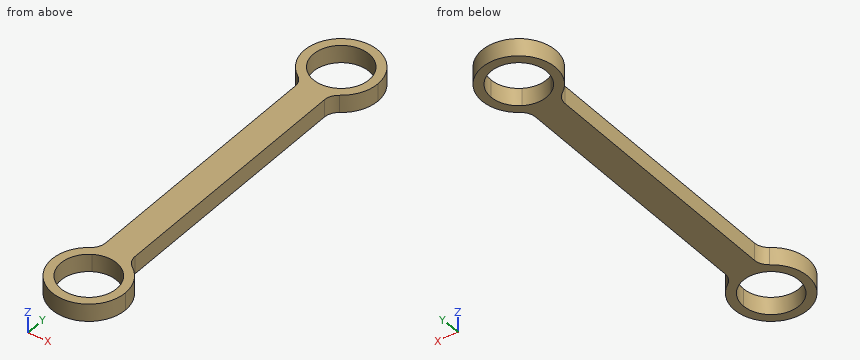
from build123d import *

# Parameters (mm, degrees)
SALIENTE_EXTRUIR1_DEPTH = 6
REDONDEO1_R             = 5


with BuildPart() as part:
    # Croquis1 → Saliente-Extruir1 (new body)
    with BuildSketch(Plane.XY):
        with BuildLine():
            ThreePointArc((-5, 103.543560763), (0, 102.5), (5, 103.543560763))
            Line((5, 103.543560763), (5, 106.922252789))
            ThreePointArc((5, 106.922252789), (0, 105.5), (-5, 106.922252789))
            Line((-5, 106.922252789), (-5, 103.543560763))
        make_face()
        with BuildLine():
            Line((5, 106.922252789), (5, 103.543560763))
            ThreePointArc((5, 103.543560763), (10.458250332, 108.153468031), (12.5, 115))
            ThreePointArc((12.5, 115), (-6.846531969, 125.458250332), (-5, 103.543560763))
            Line((-5, 103.543560763), (-5, 106.922252789))
            ThreePointArc((-5, 106.922252789), (-4.623310502, 123.299096336), (9.5, 115))
            ThreePointArc((9.5, 115), (8.299096336, 110.376689498), (5, 106.922252789))
        make_face()
        with BuildLine():
            ThreePointArc((-5, 11.456439237), (0, 12.5), (5, 11.456439237))
            Line((5, 11.456439237), (5, 103.543560763))
            ThreePointArc((5, 103.543560763), (0, 102.5), (-5, 103.543560763))
            Line((-5, 103.543560763), (-5, 11.456439237))
        make_face()
        with BuildLine():
            ThreePointArc((-5, 8.077747211), (0, 9.5), (5, 8.077747211))
            Line((5, 8.077747211), (5, 11.456439237))
            ThreePointArc((5, 11.456439237), (0, 12.5), (-5, 11.456439237))
            Line((-5, 11.456439237), (-5, 8.077747211))
        make_face()
        with BuildLine():
            Line((5, 11.456439237), (5, 8.077747211))
            ThreePointArc((5, 8.077747211), (8.299096336, 4.623310502), (9.5, 0))
            ThreePointArc((9.5, 0), (-4.623310502, -8.299096336), (-5, 8.077747211))
            Line((-5, 8.077747211), (-5, 11.456439237))
            ThreePointArc((-5, 11.456439237), (-6.846531969, -10.458250332), (12.5, 0))
            ThreePointArc((12.5, 0), (10.458250332, 6.846531969), (5, 11.456439237))
        make_face()
    extrude(amount=SALIENTE_EXTRUIR1_DEPTH)

    # Redondeo1
    redondeo1_edges = [part.edges().sort_by_distance(p)[0] for p in [
        (-5, 11.456439237, 3),
        (-5, 103.543560763, 3),
        (5, 103.543560763, 3),
        (5, 11.456439237, 3),
    ]]
    fillet(redondeo1_edges, radius=REDONDEO1_R)


solid = part.part
Input: part model. Units: mm. Frame: model coordinates. Give positions to 0.01 mm unless a question says otherwise; leave off trailing zeros. Order: outer loops, then holes, each group sorted by start corner. A loop starts at its lowest first (then second) coordinate and runs counter-clockwise, first axis right, second up. Notation, with made-up numbers: (55.5, -17) - (77.5, -17) arc R10 ccw to (77.5, 0) - close; hole circle Ø7 at (57.25, 86.25). An arc over 180 degrees is marked (long way). Write each question's results on one line, items separated by ' | '.
Item 1: Contact query for flat-ended pins moving along their axis: pin 1 Ø3 at (y, z) = (71.5, 4.5) entering from +X; pin 2 Ø10 at (x, y) = (3, 6.5) entering from -Z; pin 3 Ø3 at (x, z) = (-6, 4.5) entering from -Y; pin 4 Ø1.5 at (y, z) = (103.5, 3.5) entering from -X. Output: stop coordinate, or through.
A:
pin 1: stops at x = 5 | pin 2: stops at z = 0 | pin 3: stops at y = -11.66 | pin 4: stops at x = -6.54
Item 2: Material intervals for line 1 along Y through (x, z) = (0, 1.85); line 2 along X through (y, z) = (115, 2.8); line 3 along Y through (x, z) = (3.25, 0.4), sorted ascending.
A:
line 1: y = -12.5 to -9.5, 9.5 to 105.5, 124.5 to 127.5 | line 2: x = -12.5 to -9.5, 9.5 to 12.5 | line 3: y = -12.07 to -8.93, 8.93 to 106.07, 123.93 to 127.07
Item 3: Section C-C (y = 95). Return loops of the section in (x, z), and give its area (3 significant figures).
A:
outline: (-5, 0) - (5, 0) - (5, 6) - (-5, 6) - close | area: 60.0 mm^2
Item 4: Section A-A (x = 0). Return loops of the section in (y, z), and give its area (3 significant figures).
A:
outline: (-12.5, 0) - (-9.5, 0) - (-9.5, 6) - (-12.5, 6) - close; (9.5, 0) - (105.5, 0) - (105.5, 6) - (9.5, 6) - close; (124.5, 0) - (127.5, 0) - (127.5, 6) - (124.5, 6) - close | area: 612 mm^2
Item 5: Section B-B (z = 2.8). Return loops of the section in (x, y).
A:
outline: (-7.14, 10.26) arc R12.5 ccw (long way) to (7.14, 10.26) arc R5 cw to (5, 14.36) - (5, 100.64) arc R5 cw to (7.14, 104.74) arc R12.5 ccw (long way) to (-7.14, 104.74) arc R5 cw to (-5, 100.64) - (-5, 14.36) arc R5 cw to start; hole circle Ø19 at (0, 0); hole circle Ø19 at (0, 115)
